from build123d import *

# Parameters (mm, degrees)
SKETCH1_R            = 47.8155
BOSS_EXTRUDE1_DEPTH  = 5.08
U_BOLT_HOLES_D       = 7.9375
THREADED_ROD_HOLES_D = 7.9375


with BuildPart() as part:
    # Sketch1 → Boss-Extrude1 (new body)
    with BuildSketch(Plane(origin=(0, 0, 0), x_dir=(1, 0, 0), z_dir=(0, 1, 0))):
        Circle(SKETCH1_R)
    extrude(amount=BOSS_EXTRUDE1_DEPTH)

    # U-bolt Holes (through all)
    with Locations(Plane(origin=(0, 5.08, 0), x_dir=(1, 0, 0), z_dir=(0, 1, 0))):
        with Locations((-16.66875, 0), (16.66875, 0)):
            Hole(U_BOLT_HOLES_D / 2)

    # Threaded Rod Holes (through all)
    with Locations(Plane(origin=(0, 5.08, 0), x_dir=(1, 0, 0), z_dir=(0, 1, 0))):
        with Locations((0, 19.05), (0, -19.05)):
            Hole(THREADED_ROD_HOLES_D / 2)


solid = part.part
Model file for the job. Use its own axes, mm. Round coordinates to 2 decimals unless told otherwise and drop trailing zeros. Order: outer loops, then holes, each group sorted by start corner. A loop starts at its lowest first (then second) coordinate and runs counter-clockwise, first axis right, second up. Notation, with made-up numbers: M -29.75,35 L -7.75,35 A17 cw -7.75,56 Z; hole C 62,59 d5. An arc over 180 degrees is marked long. Write each question's results on one line, items separated by ' | '. Start each with the question number.
(1) Probe probe 1 along Z at (x, y) = (0, 3.05); probe 2 along Z at (x, y) = (-2.5, 1.65); probe 3 along X at (y, z) = (0.2, 17). List the from-to ranges inside material, lowest first. Write a range as from..to.
(2) Drop flat-ended pins along their axis: pin 1 (9 mm diameter, centred on x = 0, z = -19.05, fed in from +Y); pin 2 (5 mm diameter, centred on x = -16.67, z = 0, fed in from -Y); pin 3 (2 mm diameter, centred on y = 2.5, z = -2.5, fed in from -X); pin 4 (1 mm diameter, centred on y = 1, z = -10.5, fed in from +X). Give the stop position or say it passes through.
(3) Two-plate mould, pull along Z, no slides. Class faces 1 (the face through (-10.365, 2.504, 46.678)), 2 (the face through (-1, 5.08, -1)), 3 (the face through (-20.335, 2.504, 1.52)): pulls with the +Z half, pulls with the -Z half, needs draft (parallel to the pull), parting line crosses it, or undercut.
(4) Saw through at C-C, the plane z = -19.05. Give the cut face in (x, y), then the cut area to 3 significant figures.
(5) Saw through at D-D, the plane y = 3.8. Give the cut face in (x, z), then the cut area to 3 significant figures.
(6) Saw through at B-B, the plane x = 0. Give the cut face in (y, z).
(7) Saw through at A-A, the plane z = 0. Give the cut face in (x, y), then the cut area to 3 significant figures.
Established:
1) probe 1: z = -47.82..-23.02, -15.08..15.08, 23.02..47.82 | probe 2: z = -47.75..-22.13, -15.97..15.97, 22.13..47.75 | probe 3: x = -44.69..-3.4, 3.4..44.69
2) pin 1: stops at y = 5.08 | pin 2: passes through | pin 3: stops at x = -47.79 | pin 4: stops at x = 46.76
3) face 1: parting line crosses it | face 2: needs draft | face 3: undercut
4) outline: M -43.86,0 L -3.97,0 L -3.97,5.08 L -43.86,5.08 Z; M 3.97,0 L 43.86,0 L 43.86,5.08 L 3.97,5.08 Z | area: 405 mm^2
5) outline: C 0,0 d95.63; hole C -16.67,0 d7.94; hole C 0,-19.05 d7.94; hole C 0,19.05 d7.94; hole C 16.67,0 d7.94 | area: 6,980 mm^2
6) outline: M 0,-47.82 L 5.08,-47.82 L 5.08,-23.02 L 0,-23.02 Z; M 0,-15.08 L 5.08,-15.08 L 5.08,15.08 L 0,15.08 Z; M 0,23.02 L 5.08,23.02 L 5.08,47.82 L 0,47.82 Z
7) outline: M -47.82,0 L -20.64,0 L -20.64,5.08 L -47.82,5.08 Z; M -12.7,0 L 12.7,0 L 12.7,5.08 L -12.7,5.08 Z; M 20.64,0 L 47.82,0 L 47.82,5.08 L 20.64,5.08 Z | area: 405 mm^2
